Geometry check sheet. Reference: drawing and pictorial views, mm from the part's lowest x, y, z. A direction names the side the tool comes from. Coordinates: 2 decimals unless noted, no trailing zeros. Order: outer loops, then holes, each group sorted by start corner. A loop starts at its lowest first (then second) coordinate and runs counter-clockwise, first axis right, second up. Notation, with made-up numbers: M -29.75,19 L -10.75,19 A29 ccw -10.75,54 Z; hole C 48.25,86 d2. An arc over 180 degrees is marked long. Return JSON: item names as keys, results as strings.
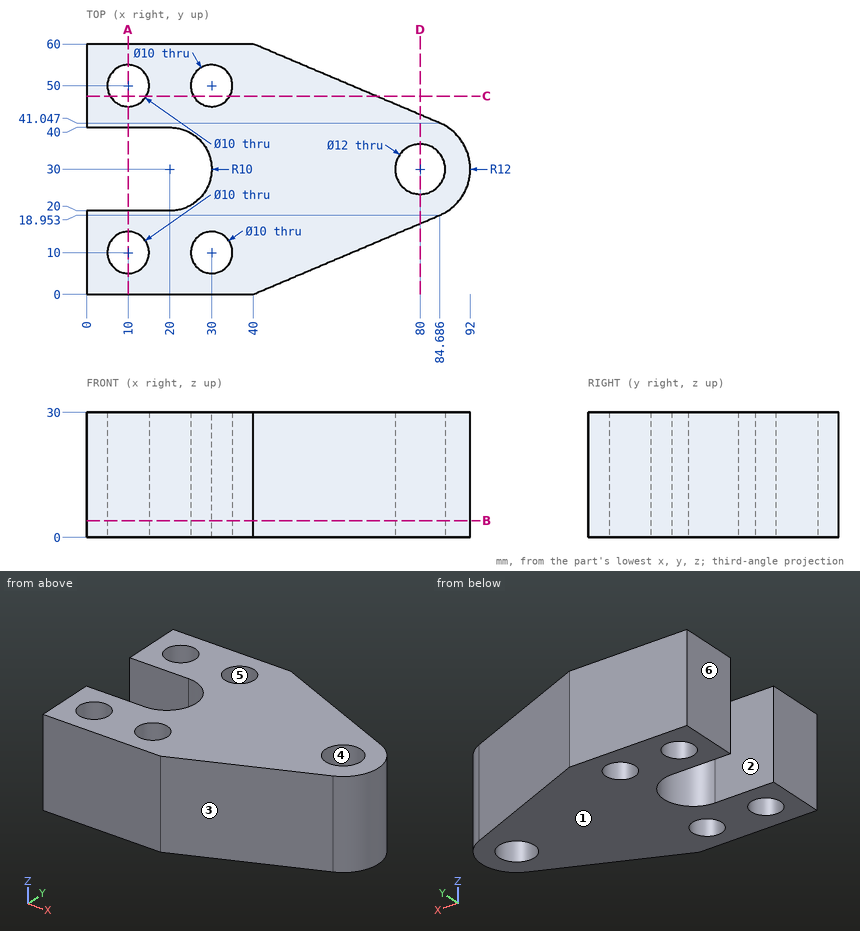
Q1. Go/stop test with flat-tipped pins: pin 1 (7 mm diameter, centred on x = 80, y = 30, fed in from -Z); pin 2 (8 mm diameter, centred on x = 68.5, z = 18.5, fed in from +Y); pin 3 (4 mm diameter, centred on x = 51.5, z = 8.5, fed in from -Y); pin 4 (5 mm diameter, centred on x = 77, z = 25, fed in from +Y). Record where each tip stops, or that it passes through.
Values:
{"pin 1": "through", "pin 2": "y = 49.61", "pin 3": "y = 4.03", "pin 4": "y = 45.37"}
Q2. Cross-section at D-D, the plane x = 80. Record the boundary of the cut face in (y, z) (1 decimal), and give its area (3 significant figures).
Values:
{"outline": "M 17,0 L 24,0 L 24,30 L 17,30 Z; M 36,0 L 43,0 L 43,30 L 36,30 Z", "area": "422 mm^2"}
Q3. Tool access check on the marked faces 1 and 2. Record the directions out of +Z, -Z, +X, -X, +Y, -Y that give a thin tool (end or side, any length) a straight path to the whole face; none if there is none.
Values:
{"face 1": "-Z, +X, -X, +Y, -Y", "face 2": "+Z, -Z, -X"}
Q4. Cross-section at A-A, the plane x = 10. Record the boundary of the cut face in (y, z), and give its area (3 significant figures).
Values:
{"outline": "M 0,0 L 5,0 L 5,30 L 0,30 Z; M 15,0 L 20,0 L 20,30 L 15,30 Z; M 40,0 L 45,0 L 45,30 L 40,30 Z; M 55,0 L 60,0 L 60,30 L 55,30 Z", "area": "600 mm^2"}
Q5. Cross-section at B-B, the plane z = 4. Record the boundary of the cut face in (x, y) (1 decimal), and give its area (3 significant figures).
Values:
{"outline": "M 0,0 L 40,0 L 84.7,19 A12 ccw 84.7,41 L 40,60 L 0,60 L 0,40 L 20,40 A10 cw 20,20 L 0,20 Z; hole C 10,10 d10; hole C 10,50 d10; hole C 30,10 d10; hole C 30,50 d10; hole C 80,30 d12", "area": "3,370 mm^2"}
Q6. Material ranges on line 1 along Y through (x, z) = (19, 21.75); line 2 along Y through (x, z) = (5.5, 19) (1 decimal); line 3 along Y through (x, z) = (33, 28), recorded low to high.
Values:
{"line 1": "0 to 20, 40 to 60", "line 2": "0 to 7.8, 12.2 to 20, 40 to 47.8, 52.2 to 60", "line 3": "0 to 6, 14 to 46, 54 to 60"}
Q7. Cross-section at C-C, the plane y = 47.5. Record the boundary of the cut face in (x, z), and give its area (3 significant figures).
Values:
{"outline": "M 0,0 L 5.67,0 L 5.67,30 L 0,30 Z; M 14.33,0 L 25.67,0 L 25.67,30 L 14.33,30 Z; M 34.33,0 L 69.47,0 L 69.47,30 L 34.33,30 Z", "area": "1,560 mm^2"}
Q8. Draft check along X on the marked faces 3, 4, 5 and 6. Enter one of: pulls with the +X half, pulls with the -X half, needs draft (parallel to the pull), parting line crosses it, or undercut.
Values:
{"face 3": "pulls with the +X half", "face 4": "undercut", "face 5": "undercut", "face 6": "pulls with the -X half"}
